Geometry: final body of the model. Coordinates: model frame, mm. A direction names the side the tool comes from. Give positions to 0.01 mm unless a question says otherwise; leave off trailing zeros. Write each loop counter-clockwise with the first axis right and the second up, starting at its lowest first coordinate (ties: lowest second). Pieces come first, ordered by that corner, then holes.
```python
from build123d import *

# Parameters (mm, degrees)
F0_W         = 88.9
F0_H         = 127
F1_DEPTH     = 88.9
F3_DEPTH     = 5.08
F4_DEPTH     = 25.4
F2_W         = 78.3582460135
F2_H         = 44.45
F5_DEPTH     = 120.65
F6_DEPTH     = 25.4
F7_R         = 9.4165633134
F8_DEPTH     = 38.1
F9_DEPTH     = 38.1
F10_DEPTH    = 25.4
F11_DEPTH    = 101.6
F12_R        = 3.7821151403
F13_DEPTH    = 25.4
F14_R        = 8.3394092173
F15_DEPTH    = 25.4
F16_R        = 6.9968499513
F17_DEPTH    = 25.4
F18_R        = 3.8523221967
F19_DEPTH    = 25.4
F20_R        = 9.4524039115
F21_DEPTH    = 25.4
F22_R        = 3.8935430456
F22_R_2      = 2.5048426579
F22_R_3      = 5.3475780775
F22_R_4      = 3.5866360784
F22_R_5      = 3.0785479475
F23_DEPTH    = 25.4
F24_R        = 10.2887517637
F24_R_2      = 3.7572197848
F24_R_3      = 4.8207100709
F24_R_4      = 7.7084596518
F24_R_5      = 4.0689133859
F24_R_6      = 8.3104077663
F24_R_7      = 5.128893449
F24_R_8      = 5.5582930393
F24_R_9      = 3.9454288103
F24_R_10     = 3.6254323416
F24_R_11     = 3.933516476
F25_DEPTH    = 25.4
F27_DEPTH    = 60.96
F28_W        = 33.8233187795
F28_H        = 48.4882295132
F29_DEPTH    = 25.4
F30_T1_DEPTH = 21.59
F31_R        = 12.7015512299
F32_DEPTH    = 25.4


# Not quite as in the source:
# - a fillet or chamfer that OpenCascade refuses, or shapes differently, is made with other operations: its cross-section is extruded or revolved along the edge and cut away or added


with BuildPart() as f1:
    # F0 (on Top) → F1 (new body)
    with BuildSketch(Plane.XY):
        with Locations((44.45, 63.5)):
            Rectangle(F0_W, F0_H)
    extrude(amount=F1_DEPTH)

    # F3 (add): a face of the model
    f3_faces = [f1.faces().sort_by_distance(p)[0] for p in [
        (44.45, 63.5, 0),
    ]]
    extrude(f3_faces, amount=F3_DEPTH)

    # F4 (add): a face of the model
    f4_faces = [f1.faces().sort_by_distance(p)[0] for p in [
        (44.45, 127, 41.91),
    ]]
    extrude(f4_faces, amount=F4_DEPTH)

    # F2 (on face) → F5 (cut)
    with BuildSketch(Plane.XZ):
        with Locations((44.9183965102, 22.225)):
            Rectangle(F2_W, F2_H)
    extrude(amount=-F5_DEPTH, mode=Mode.SUBTRACT)

    # F6 (cut): a face of the model
    f6_faces = [f1.faces().sort_by_distance(p)[0] for p in [
        (44.45, 152.4, 41.91),
    ]]
    extrude(f6_faces, amount=-F6_DEPTH, mode=Mode.SUBTRACT)

    # F7 (on face) → F8 (cut)
    with BuildSketch(Plane.XY.offset(88.9)):
        with Locations((23.3609545976, 24.8096976429)):
            Circle(F7_R)
    extrude(amount=-F8_DEPTH, mode=Mode.SUBTRACT)

    # F9 (add): a face of the model
    f9_faces = [f1.faces().sort_by_distance(p)[0] for p in [
        (44.9835020735, 64.4787714966, 88.9),
    ]]
    extrude(f9_faces, amount=F9_DEPTH)

    # F10 (add): a face of the model
    f10_faces = [f1.faces().sort_by_distance(p)[0] for p in [
        (44.9183965102, 120.65, 22.225),
    ]]
    extrude(f10_faces, amount=F10_DEPTH)

    # F11 (cut): a face of the model
    f11_faces = [f1.faces().sort_by_distance(p)[0] for p in [
        (44.9183965102, 95.25, 22.225),
    ]]
    extrude(f11_faces, amount=-F11_DEPTH, mode=Mode.SUBTRACT)

    # F12 (on face) → F13 (cut)
    with BuildSketch(Plane(origin=(0, 0, 0), x_dir=(0, -1, 0), z_dir=(-1, 0, 0))):
        with Locations((-20.8959858865, 22.2413502634)):
            Circle(F12_R)
    extrude(amount=-F13_DEPTH, mode=Mode.SUBTRACT)

    # F14 (on face) → F15 (cut)
    with BuildSketch(Plane(origin=(0, 0, 0), x_dir=(0, -1, 0), z_dir=(-1, 0, 0))):
        with Locations((-106.0243174434, 31.2219746411)):
            Circle(F14_R)
    extrude(amount=-F15_DEPTH, mode=Mode.SUBTRACT)

    # F16 (on face) → F17 (cut)
    with BuildSketch(Plane(origin=(0, 0, 0), x_dir=(0, -1, 0), z_dir=(-1, 0, 0))):
        with Locations((-75.6411701441, 14.8054044694)):
            Circle(F16_R)
    extrude(amount=-F17_DEPTH, mode=Mode.SUBTRACT)

    # F18 (on face) → F19 (cut)
    with BuildSketch(Plane(origin=(0, 0, 0), x_dir=(0, -1, 0), z_dir=(-1, 0, 0))):
        with Locations((-59.9940270185, 33.8436961174)):
            Circle(F18_R)
    extrude(amount=-F19_DEPTH, mode=Mode.SUBTRACT)

    # F20 (on face) → F21 (cut)
    with BuildSketch(Plane.YZ.offset(5.7392735034)):
        with Locations((38.390211761, 14.1541231424)):
            Circle(F20_R)
    extrude(amount=-F21_DEPTH, mode=Mode.SUBTRACT)

    # F22 (on face) → F23 (cut)
    with BuildSketch(Plane.YZ.offset(5.7392735034)):
        with Locations((103.7926003337, 9.5047177747)):
            Circle(F22_R)
        with Locations((29.4643323869, 32.8702926636)):
            Circle(F22_R_2)
        with Locations((9.4724670053, 9.5047177747)):
            Circle(F22_R_3)
        with Locations((47.9597039521, 26.7663411796)):
            Circle(F22_R_4)
        with Locations((75.3153562546, 34.4844758511)):
            Circle(F22_R_5)
    extrude(amount=-F23_DEPTH, mode=Mode.SUBTRACT)

    # F24 (on face) → F25 (cut)
    with BuildSketch(Plane(origin=(84.0975195169, 0, 0), x_dir=(0, -1, 0), z_dir=(-1, 0, 0))):
        with Locations((-100.267700851, 32.3584228754)):
            Circle(F24_R)
        with Locations((-89.9443402886, 16.390549019)):
            Circle(F24_R_2)
        with Locations((-114.4196018577, 6.8739750423)):
            Circle(F24_R_3)
        with Locations((-42.5033308566, 35.6052704155)):
            Circle(F24_R_4)
        with Locations((-74.3665918708, 29.6205114573)):
            Circle(F24_R_5)
        with Locations((-47.0789894462, 15.7656241208)):
            Circle(F24_R_6)
        with Locations((-7.5106075965, 16.2924602628)):
            Circle(F24_R_7)
        with Locations((-24.5902761817, 24.7659608722)):
            Circle(F24_R_8)
        with Locations((-10.5220889673, 38.1775014102)):
            Circle(F24_R_9)
        with Locations((-75.9231299162, 9.4177098945)):
            Circle(F24_R_10)
        with Locations((-25.1116491854, 10.8577311039)):
            Circle(F24_R_11)
    extrude(amount=-F25_DEPTH, mode=Mode.SUBTRACT)

    # F26 (on face) → F27 (cut)
    with BuildSketch(Plane(origin=(0, 0, 44.45), x_dir=(1, 0, 0), z_dir=(0, 0, -1))):
        Polygon((84.0975195169, 0), (44.9183965102, 0), (44.9183965102, -43.4251762927), (5.7392735034, -43.4251762927), (5.7392735034, -127), (84.0975195169, -127), align=None)
    extrude(amount=-F27_DEPTH, mode=Mode.SUBTRACT)

    # F28 (on face) → F29 (cut)
    with BuildSketch(Plane.XY.offset(127)):
        with Locations((29.9662053585, 90.6256511807)):
            Rectangle(F28_W, F28_H)
    extrude(amount=-F29_DEPTH, mode=Mode.SUBTRACT)

    # F30: fillet of radius 17.78 on 4 edges, made by hand

    # F30_s2 → F30_t1 (join)
    with BuildSketch(Plane.XY.offset(105.41)):
        with BuildLine():
            ThreePointArc((29.0978647482, 66.3815364242), (41.6702233177, 71.5891778547), (46.8778647482, 84.1615364242))
            Line((46.8778647482, 84.1615364242), (46.8778647482, 66.3815364242))
            Line((46.8778647482, 66.3815364242), (29.0978647482, 66.3815364242))
        make_face()
        with BuildLine():
            ThreePointArc((13.0545459688, 84.1615364242), (18.2621873993, 71.5891778547), (30.8345459688, 66.3815364242))
            Line((30.8345459688, 66.3815364242), (13.0545459688, 66.3815364242))
            Line((13.0545459688, 66.3815364242), (13.0545459688, 84.1615364242))
        make_face()
        with BuildLine():
            ThreePointArc((29.0978647482, 114.8697659373), (41.6702233177, 109.6621245068), (46.8778647482, 97.0897659373))
            Line((46.8778647482, 97.0897659373), (46.8778647482, 114.8697659373))
            Line((46.8778647482, 114.8697659373), (29.0978647482, 114.8697659373))
        make_face()
        with BuildLine():
            ThreePointArc((30.8345459688, 114.8697659373), (18.2621873993, 109.6621245068), (13.0545459688, 97.0897659373))
            Line((13.0545459688, 97.0897659373), (13.0545459688, 114.8697659373))
            Line((13.0545459688, 114.8697659373), (30.8345459688, 114.8697659373))
        make_face()
    extrude(amount=F30_T1_DEPTH)

    # F31 (on face) → F32 (cut)
    with BuildSketch(Plane.XY.offset(127)):
        with Locations((66.893927753, 92.3067107797)):
            Circle(F31_R)
    extrude(amount=-F32_DEPTH, mode=Mode.SUBTRACT)


solid = f1.part
```
Item 1: Section C-C, the plane x = 21.5. Return the cut outline in (y, z).
Found:
outline: (0, -5.08) - (127, -5.08) - (127, 0) - (0, 0) - close; (0, 44.45) - (43.43, 44.45) - (43.43, 105.41) - (69.03, 105.41) - (69.03, 127) - (34.04, 127) - (34.04, 50.8) - (15.58, 50.8) - (15.58, 127) - (0, 127) - close; (112.22, 105.41) - (127, 105.41) - (127, 127) - (112.22, 127) - close
Item 2: Section D-D, the plane x = 8.5. Return the cut outline in (y, z), plus the area to 3 significant figures.
Found:
outline: (0, -5.08) - (127, -5.08) - (127, 0) - (0, 0) - close; (0, 44.45) - (43.43, 44.45) - (43.43, 105.41) - (127, 105.41) - (127, 127) - (0, 127) - close
area: 6,030 mm2
Item 3: Section B-B, the plane z = 53. Return the cut outline in (x, y).
Found:
outline: (0, 0) - (44.92, 0) - (44.92, 43.43) - (5.74, 43.43) - (5.74, 127) - (0, 127) - close; (84.1, 0) - (88.9, 0) - (88.9, 127) - (84.1, 127) - close; hole circle Ø18.83 at (23.36, 24.81)
Item 4: Line query: L1, parallel to Z at x = 76, y = 30.5; L2, parallel to Z at x = 41.5, y = 35.5; L3, parallel to X at y = 19, z = 71.5. Output: solid intervals per line, ascending.
Found:
L1: z = -5.08 to 0, 105.41 to 127
L2: z = -5.08 to 0, 44.45 to 127
L3: x = 0 to 15.95, 30.77 to 44.92, 84.1 to 88.9
Item 5: Reachability of faces 4 (the face through (84.098, 64, 52)), 5 (the face through (23, 25, 50.8)), 6 (the face through (54, 64, 105.41)), 7 (the face through (86.5, 48.2, 24)), 8 (the face through (2.91, 51.27, 25.39)) from +Z, -Z, +X, -X, +Y, -Y: full face, straight path, thin tool, end or side. Return the list, or none.
Found:
face 4: +Y, -Y
face 5: +Z
face 6: +Y
face 7: +X
face 8: -X
Item 6: Section A-A, the plane x = 50. Return the cut outline in (y, z).
Found:
outline: (0, -5.08) - (127, -5.08) - (127, 0) - (0, 0) - close; (0, 105.41) - (127, 105.41) - (127, 127) - (0, 127) - close
Item 7: Pull-direction query (Y, two-part tool) for faces 1 (the face through (44, 63, -5.08)), 2 (the face through (24, 0, 75)), 3 (the face through (54.205, 92.865, 116.356)); classes: +Y half, -Y half, draft (parallel to the pull), parting line (faces both ways), or undercut.
Found:
face 1: draft
face 2: -Y half
face 3: undercut
Item 8: Pin query (flat end, axial travel): pin 1 Ø17 at (y, z) = (38.39, 14.15) entering from -X; pin 2 Ø6.5 at (y, z) = (74.37, 29.62) entering from +X; pin 3 Ø11.5 at (x, y) = (23.36, 24.81) entering from +Z. Return the tip coordinate at first contact, or that it passes through.
Found:
pin 1: stops at x = 84.1
pin 2: stops at x = 5.74
pin 3: stops at z = 50.8
